```python
from build123d import *

# Parameters (mm, degrees)
SKETCH_1_R          = 16
EXTRUDE_1_DEPTH     = 25
FILLET_1_R          = 2
SKETCH_3_R          = 2.5
CUT_EXTRUDE_1_DEPTH = 30
EXTRUDE_START       = -8
SKETCH_4_R          = 16
SKETCH_4_R_2        = 14
EXTRUDE_2_DEPTH     = 8


with BuildPart() as part:
    # 草图1 → 凸台-拉伸1 (new body)
    with BuildSketch(Plane.XY):
        Polygon((-22.5, 50), (22.5, 50), (22.5, -85), (62.5, -85), (62.5, -110), (22.5, -110), (-22.5, -110), (-62.5, -110), (-62.5, -85), (-22.5, -85), align=None)
        with Locations((0, 30)):
            Circle(SKETCH_1_R, mode=Mode.SUBTRACT)
    extrude(amount=EXTRUDE_1_DEPTH)

    # 圆角1
    fillet_1_edges = [part.edges().sort_by_distance(p)[0] for p in [
        (-22.5, -85, 12.5),
        (22.5, -85, 12.5),
    ]]
    fillet(fillet_1_edges, radius=FILLET_1_R)

    # 草图3 → 切除-拉伸1 (cut)
    with BuildSketch(Plane(origin=(0, -85, 0), x_dir=(1, 0, 0), z_dir=(0, 1, 0))):
        with Locations(Location((-45, -12.5, 0), (0, 0, 270))):
            Circle(SKETCH_3_R)
        with Locations(Location((45, -12.5, 0), (0, 0, 270))):
            Circle(SKETCH_3_R)
    extrude(amount=-CUT_EXTRUDE_1_DEPTH, mode=Mode.SUBTRACT)

    # 草图4 → 凸台-拉伸2 (add)
    with BuildSketch(Plane.XY.offset(25).offset(EXTRUDE_START)):
        with Locations((0, 30)):
            Circle(SKETCH_4_R)
        with Locations((0, 30)):
            Circle(SKETCH_4_R_2, mode=Mode.SUBTRACT)
    extrude(amount=EXTRUDE_2_DEPTH)


solid = part.part
```
The model under review builds one solid part; all positions refer to its coordinate system, in mm. A direction names the side the tool comes from. Round coordinates to 2 decimals unless told otherwise and drop trailing zeros. Loops run counter-clockwise (first coordinate to the right, second up) from the corner with the lowest first, then second, coordinate; pieces in that order, holes last. Notation, with made-up numbers: M 72,17.5 L 86,17.5 A21 cw 86,48.5 Z; hole C 19.25,73.25 d3. An arc over 180 degrees is marked long. Write item = value, one per line.
Item 1: Take a section at C-C on y = 30. Write out the cut boundary in (x, z), then the cut area to 3 significant figures.
Return value:
outline = M -22.5,0 L -16,0 L -16,17 L -14,17 L -14,25 L -22.5,25 Z; M 14,17 L 16,17 L 16,0 L 22.5,0 L 22.5,25 L 14,25 Z
area = 357 mm2
Item 2: Take a section at B-B on x = 45. Write out the cut boundary in (y, z), then the cut area to 3 significant figures.
Return value:
outline = M -110,0 L -85,0 L -85,10 L -110,10 Z; M -110,15 L -85,15 L -85,25 L -110,25 Z
area = 500 mm2
Item 3: Insertion check: P1, Ø3, axis at y = -41.5, z = 21, coming from the -X side; P2, Ø16, axis at x = 1, y = 27, coming from the -Z side; P3, Ø12.5, axis at x = -48.5, z = 16.5, coming from the +Y side; P4, Ø12.5, axis at y = -24.5, z = 15, coming from the +X side. Each pin has a flat end and moves straight along its axis. Give the tip position at first contact, or say it passes through.
Return value:
P1 = -22.5
P2 = through
P3 = -85
P4 = 22.5
Item 4: Machinability: for faces 1 (the flat face through (43, -85, 10)), 2 (the flat face through (-1, -47, 25)), 3 (the flat face through (-44, -85, 10)), 4 (the flat face through (-0.07, 15.85, 17)), which of the approach directions +Z, -Z, +X, -X, +Y, -Y give a long, thin tool a straight path to every point of the face, cutting with its end or side? Answer none if there is none.
Return value:
face_1 = +Z, -Z, +X, +Y
face_2 = +Z, +X, -X, +Y, -Y
face_3 = +Z, -Z, -X, +Y
face_4 = -Z
Item 5: For line 1 (X direction, y = -92.5, z = 12.5); line 2 (Y direction, x = 0, z = 20.5); line 3 (X direction, y = -22, z = 21.5), list the stretches that pass through material, from the lowest coordinate up. Write a range as [from, to].
Return value:
line_1 = [-62.5, -47.5], [-42.5, 42.5], [47.5, 62.5]
line_2 = [-110, 16], [44, 50]
line_3 = [-22.5, 22.5]
Item 6: Take a section at A-A on z = 12.5. Write out the cut boundary in (x, y).
Return value:
outline = M -62.5,-110 L -47.5,-110 L -47.5,-85 L -62.5,-85 Z; M -42.5,-110 L 42.5,-110 L 42.5,-85 L 24.5,-85 A2 cw 22.5,-83 L 22.5,50 L -22.5,50 L -22.5,-83 A2 cw -24.5,-85 L -42.5,-85 Z; M 47.5,-110 L 62.5,-110 L 62.5,-85 L 47.5,-85 Z; hole C 0,30 d32
Item 7: Take a section at D-D on z = 20.25. Write out the cut boundary in (x, y), then the cut area to 3 significant figures.
Return value:
outline = M -62.5,-110 L 62.5,-110 L 62.5,-85 L 24.5,-85 A2 cw 22.5,-83 L 22.5,50 L -22.5,50 L -22.5,-83 A2 cw -24.5,-85 L -62.5,-85 Z; hole C 0,30 d28
area = 8,590 mm2
Item 8: The part is to be moulded in two halves that separate along Y. For faces 5 (the flat face through (0, 50, 12)), 6 (the cylindrical face through (-3.47, 14.38, 8.38)), 7 (the flat face through (-22.5, -17, 12)), say which applies: released by +Y, released by -Y, zero draft, split by the parting line, or undercut.
Return value:
face_5 = released by +Y
face_6 = undercut
face_7 = zero draft
